Check sheet for the modelled part. Datum: model origin and axes. Units: mm. Face numbers are marked on the shaded views. A direction names the side the tool comes from. Round coordinates to 2 decimals unless told otherwise and drop trailing zeros. Write each loop counter-clockwise with the first axis right and the second up, starting at its lowest first coordinate (ties: lowest second). Pieces come first, ordered by that corner, then holes. Notation, with made-up numbers: (12, -26.75) -> (50, -26.75) arc R33 cw to (50, 5.25) -> close; hole circle Ø4 at (65.5, 74.5). An arc over 180 degrees is marked (long way). One line per item, written item: value.
from build123d import *

# Parameters (mm, degrees)
SKETCH1_R           = 3.2000000000000006
SKETCH1_R_2         = 3.2000000000000037
SKETCH1_R_3         = 1.2500000000000047
BOSS_EXTRUDE1_DEPTH = 10
SKETCH1_7_R         = 1.2500000000000122
BOSS_EXTRUDE2_DEPTH = 10
FILLET1_R           = 10
FILLET2_R           = 2
FILLET3_R           = 2


with BuildPart() as part:
    # Sketch1 → Boss-Extrude1 (new body)
    with BuildSketch(Plane(origin=(0, 0, 0), x_dir=(1, 0, 0), z_dir=(0, 1, 0))):
        with BuildLine():
            Line((-9.148889755102248, 0.2602426865805545), (73.5491158361503, 87.21448278577964))
            ThreePointArc((73.5491158361503, 87.21448278577964), (84.15238119180354, 87.48049744252629), (84.41839584855015, 76.87723208687311))
            Line((84.41839584855015, 76.87723208687311), (1.7203902572976446, -10.077008012326013))
            ThreePointArc((1.7203902572976446, -10.077008012326013), (-8.882875098355584, -10.343022669072676), (-9.148889755102248, 0.2602426865805545))
        make_face()
        with Locations(Location((-3.7142497489023008, -4.908382662872731, 0), (0, 0, 270))):
            Circle(SKETCH1_R, mode=Mode.SUBTRACT)
        with Locations(Location((41.769653326286615, 42.91644939168677, 0), (0, 0, 270))):
            Circle(SKETCH1_R_2, mode=Mode.SUBTRACT)
        with Locations(Location((31.432402627380036, 32.047169379286885, 0), (0, 0, 270))):
            Circle(SKETCH1_R_3, mode=Mode.SUBTRACT)
    extrude(amount=-BOSS_EXTRUDE1_DEPTH)

    # Sketch1<7> → Boss-Extrude2 (add)
    with BuildSketch(Plane(origin=(0, 0, 0), x_dir=(1, 0, 0), z_dir=(0, 1, 0))):
        with BuildLine():
            Line((62.691064287297834, 75.79759776372697), (55.55645800762751, 68.29579330036361))
            Line((55.55645800762751, 68.2957933003636), (81.85576990080861, 25.27333022283284))
            ThreePointArc((81.85576990080861, 25.27333022283284), (88.7296482404513, 23.61507916470229), (90.38789929858186, 30.488957504344977))
            Line((90.38789929858186, 30.488957504344977), (62.69106428729781, 75.79759776372696))
        make_face()
        with Locations(Location((86.12183459969525, 27.881143863588914, 0), (0, 0, 270))):
            Circle(SKETCH1_7_R, mode=Mode.SUBTRACT)
    extrude(amount=BOSS_EXTRUDE2_DEPTH)

    # Fillet1
    fillet1_edges = [part.edges().sort_by_distance(p)[0] for p in [
        (59.12376114746267, 10, -72.04669553204529),
    ]]
    fillet(fillet1_edges, radius=FILLET1_R)

    # Fillet2
    # the kernel refuses this fillet: 2 mm, written as the material it adds along each edge
    with BuildSketch(Plane(origin=(52.94864436687145, 0, -72.56185799925024), x_dir=(-0.853212939777324, 0, 0.5215627281512133), z_dir=(0.5215627281512133, 0, 0.853212939777324))) as fillet2_piece_1_section:
        with BuildLine():
            CenterArc((FILLET2_R, -FILLET2_R), FILLET2_R, 90, 90)
            Line((-6.06e-15, -FILLET2_R), (0, 0))
            Line((0, 0), (FILLET2_R, 0))
        make_face()
    fillet2_piece_1 = extrude(amount=25.52914270615122, mode=Mode.PRIVATE)
    fillet2_piece_1 = fillet2_piece_1 & Plane(origin=(61.097194422091576, 1.78e-15, -59.61106783019719), x_dir=(-0.7246186674933254, 0, -0.6891500465937715), z_dir=(-0.6891500465937715, 0, 0.7246186674933254)) * Cylinder(10, 60, mode=Mode.PRIVATE)
    fillet2_piece_1 = split(fillet2_piece_1, bisect_by=Plane(origin=(64.72028775955818, 0.44613502682003076, -56.16531759722836), z_dir=(-0.7246186674933262, 0, -0.6891500465937709)), keep=Keep.TOP, mode=Mode.PRIVATE)
    add(fillet2_piece_1)
    with BuildSketch(Plane(origin=(73.39829996372362, 0, -58.28186756430348), x_dir=(0.853212939777324, 0, -0.5215627281512135), z_dir=(-0.5215627281512135, 0, -0.8532129397773239))) as fillet2_piece_2_section:
        with BuildLine():
            CenterArc((FILLET2_R, -FILLET2_R), FILLET2_R, 90, 90)
            Line((0, -FILLET2_R), (0, 0))
            Line((0, 0), (FILLET2_R, 0))
        make_face()
    fillet2_piece_2 = extrude(amount=25.529142706151212, mode=Mode.PRIVATE)
    fillet2_piece_2 = fillet2_piece_2 & Plane(origin=(68.86970126476385, 1.78e-15, -67.78360381021702), x_dir=(-0.7246186674933254, 0, -0.6891500465937715), z_dir=(-0.6891500465937715, 0, 0.7246186674933254)) * Cylinder(10, 60, mode=Mode.PRIVATE)
    fillet2_piece_2 = split(fillet2_piece_2, bisect_by=Plane(origin=(72.49279460223045, 0.4461350127240334, -64.3378535772482), z_dir=(-0.7246186674933262, 0, -0.6891500465937709)), keep=Keep.TOP, mode=Mode.PRIVATE)
    add(fillet2_piece_2)

    # Fillet3
    fillet3_edges = [part.edges().sort_by_distance(p)[0] for p in [
        (67.22318318313239, 0, -58.797030031508406),
    ]]
    fillet(fillet3_edges, radius=FILLET3_R)


solid = part.part
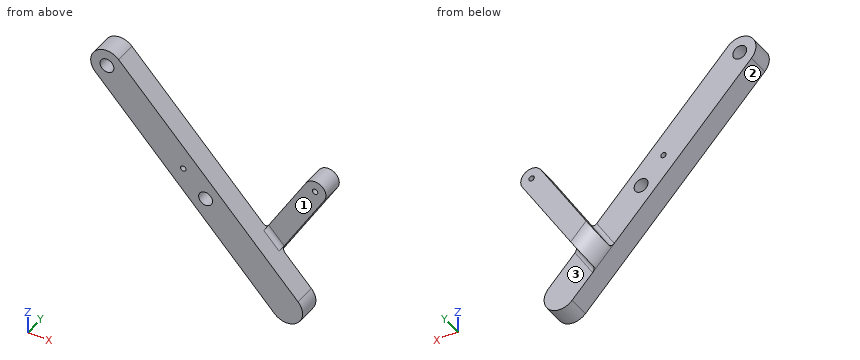
Item 1: Thickness scan on line 1 (Y direction, x = 71.5, z = -50.5); line 2 (Z direction, x = -3.5, y = -9); line 3 (Z direction, x = 31, y = -9). Record the ranges inside material, lowest first.
Answer:
line 1: y = 0 to 10
line 2: z = -6.2 to 1.72, 8.1 to 12.41
line 3: z = -42.48 to -33.22, -30.87 to -20.71
Item 2: Sectioned sample at D-D on y = -7.75. Enter the section's corners in (x, z).
Answer:
outline: (-9.15, -0.26) -> (73.55, -87.21) arc R7.5 ccw to (84.42, -76.88) -> (1.72, 10.08) arc R7.5 ccw to start; hole circle Ø6.4 at (-3.71, 4.91); hole circle Ø2.5 at (31.43, -32.05); hole circle Ø6.4 at (41.77, -42.92)
Item 3: Sectioned sample at B-B on z = 3. Enter the section's corners in (x, y), and give its area (3 significant figures).
Answer:
outline: (-10.97, -10) -> (-6.28, -10) -> (-6.28, 0) -> (-10.97, 0) -> close; (-1.15, -10) -> (8.45, -10) -> (8.45, 0) -> (-1.15, 0) -> close
area: 143 mm^2
Item 4: Tool access check on the marked faces 1, 2 and 3. Record the directions out of +Z, -Z, +X, -X, +Y, -Y that give a thin tool (end or side, any length) a straight path to the whole face; none if there is none.
Answer:
face 1: +Z, +X, -Y
face 2: -Z, -X, +Y, -Y
face 3: -Z, +X, +Y
Item 5: Depth check by flat-ended pin: P1, Ø8, axis at x = 14, y = -2.5, coming from the -Z side; P2, Ø4, axis at x = 55, z = -45, coming from the -Y side; P3, Ø10, axis at x = 12.5, y = -2.5, coming from the +Z side; P4, Ø10, axis at x = 62.5, y = 1.5, coming from the +Z side. Enter the tip coordinate at first touch or a pass-through.
Answer:
P1: stops at z = -28.81
P2: stops at y = -10
P3: stops at z = 4
P4: stops at z = -48.76
Item 6: Sectioned sample at C-C on y = 5.25. Enter the section's corners in (x, z), and give its area (3 significant figures).
Answer:
outline: (56.36, -66.98) -> (63.5, -74.48) -> (90.39, -30.49) arc R5 ccw to (81.86, -25.27) -> close; hole circle Ø2.5 at (86.12, -27.88)
area: 537 mm^2
Item 7: Sectioned sample at A-A on x = 78.5. Enter the section's corners in (y, z).
Answer:
outline: (-10, -89.53) -> (0, -89.53) -> (0, -70.65) -> (-10, -70.65) -> close; (0, -49.94) -> (10, -49.94) -> (10, -30.76) -> (0, -30.76) -> close
